Answer from the drawing. Dimensions are ordinates in mm from the lowest x, y and z of the part. Round coordinates to 2 decimals unless told otherwise and drop trailing zeros. Loops run counter-clockwise (first coordinate to the right, second up) from the corner with the lowest first, then second, coordinate; pieces in that order, holes last. Notation, with made-up numbers: (-28, 4) - (-2, 4) arc R17 ccw to (-2, 9) - close; hole circle Ø9 at (81.25, 27.25). An arc over 180 degrees is marked (long way). Use CSV: the item, a comma, the result in double quotes. Start each with the question number.
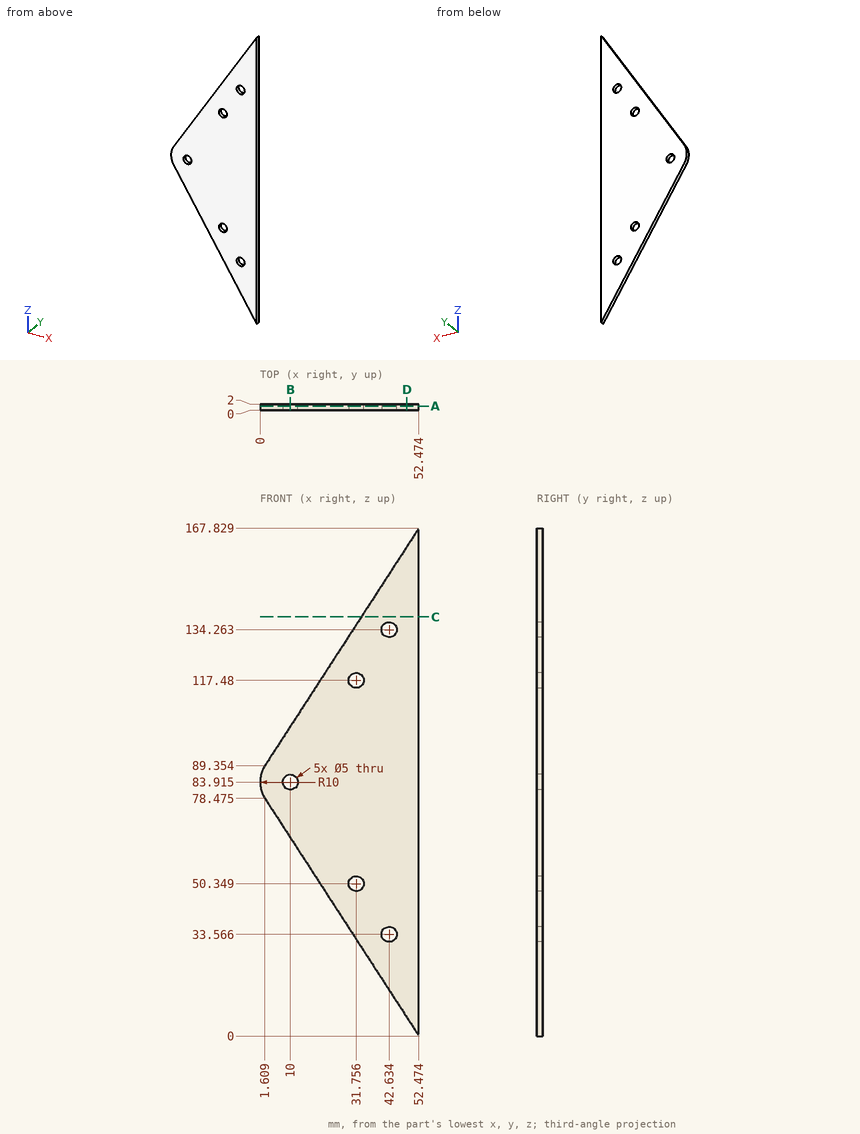
Item 1: Find the intervals of material crossed by probe 1 along Z at (x, y) = (42.5, 1.2) (1 decimal); probe 2 along X at (y, z) = (1.85, 84); probe 3 along X at (y, z) = (1.1, 84.5) (1 decimal), in increasing order. Write a range as [from, to].
Item 2: A cutting plane is placed at B-B (x = 10). Determine the outline of the cut face in (y, z) (1 decimal).
Item 3: A cutting plane is placed at D-D (x = 48.5). Determine the outline of the cut face in (y, z), plus the area to 3 significant figures.
Item 4: A cutting plane is placed at C-C (z = 138.5). Determine the outline of the cut face in (x, y).
Item 5: A cutting plane is placed at A-A (y = 1.3). Determine the outline of the cut face in (x, z) (1 decimal), plus the area to 3 significant figures.
Result sheet:
1,probe 1,"[15.4, 31.1], [36.1, 131.8], [136.8, 152.4]"
1,probe 2,"[0, 7.5], [12.5, 52.47]"
1,probe 3,"[0, 7.6], [12.4, 52.5]"
2,outline,"(0, 65.5) - (2, 65.5) - (2, 81.4) - (0, 81.4) - close; (0, 86.4) - (2, 86.4) - (2, 102.3) - (0, 102.3) - close"
3,outline,"(0, 6.13) - (2, 6.13) - (2, 161.7) - (0, 161.7) - close"
3,area,"311 mm^2"
4,outline,"(33.46, 0) - (52.47, 0) - (52.47, 2) - (33.46, 2) - close"
5,outline,"(1.6, 78.5) - (52.5, 0) - (52.5, 167.8) - (1.6, 89.4) arc R10 ccw to start; hole circle Ø5 at (10, 83.9); hole circle Ø5 at (31.8, 50.3); hole circle Ø5 at (31.8, 117.5); hole circle Ø5 at (42.6, 33.6); hole circle Ø5 at (42.6, 134.3)"
5,area,"4,460 mm^2"
